from build123d import *

# Parameters (mm, degrees)
BOSS_EXTRUDE1_DEPTH = 76.2
CUT_EXTRUDE1_DEPTH  = 10
SKETCH4_R           = 10
SKETCH4_R_2         = 12.7
CUT_EXTRUDE2_DEPTH  = 10


with BuildPart() as part:
    # Sketch2 → Boss-Extrude1 (new, symmetric)
    with BuildSketch(Plane.XY):
        with BuildLine():
            Line((-38.1, 0), (38.1, 0))
            Line((38.1, 0), (38.1, 101.6))
            Line((38.1, 101.6), (34.925, 101.6))
            ThreePointArc((34.925, 101.6), (32.67993597, 100.67006403), (31.75, 98.425))
            Line((31.75, 98.425), (31.75, 9.525))
            ThreePointArc((31.75, 9.525), (30.82006403, 7.27993597), (28.575, 6.35))
            Line((28.575, 6.35), (-34.925, 6.35))
            ThreePointArc((-34.925, 6.35), (-37.17006403, 5.42006403), (-38.1, 3.175))
            Line((-38.1, 3.175), (-38.1, 0))
        make_face()
    extrude(amount=BOSS_EXTRUDE1_DEPTH, both=True)

    # Sketch3 → Cut-Extrude1 (cut)
    with BuildSketch(Plane(origin=(38.1, 0, 0), x_dir=(0, 0, -1), z_dir=(1, 0, 0))):
        with BuildLine():
            Line((-28.25, 88.9), (-28.25, 38.1))
            ThreePointArc((-28.25, 38.1), (-31.75, 34.6), (-35.25, 38.1))
            Line((-35.25, 38.1), (-35.25, 88.9))
            ThreePointArc((-35.25, 88.9), (-31.75, 92.4), (-28.25, 88.9))
        make_face()
        with BuildLine():
            Line((28.25, 88.9), (28.25, 38.1))
            ThreePointArc((28.25, 38.1), (31.75, 34.6), (35.25, 38.1))
            Line((35.25, 38.1), (35.25, 88.9))
            ThreePointArc((35.25, 88.9), (31.75, 92.4), (28.25, 88.9))
        make_face()
        with BuildLine():
            Line((3.5, 88.9), (3.5, 38.1))
            ThreePointArc((3.5, 38.1), (0, 34.6), (-3.5, 38.1))
            Line((-3.5, 38.1), (-3.5, 88.9))
            ThreePointArc((-3.5, 88.9), (0, 92.4), (3.5, 88.9))
        make_face()
    extrude(amount=-CUT_EXTRUDE1_DEPTH, mode=Mode.SUBTRACT)

    # Sketch4 → Cut-Extrude2 (cut)
    with BuildSketch(Plane.XZ):
        with Locations(Location((0, 0, 0), (0, 0, 270))):
            Circle(SKETCH4_R)
        with Locations(Location((0, 52.5, 0), (0, 0, 270))):
            Circle(SKETCH4_R_2)
        with Locations(Location((0, -52.5, 0), (0, 0, 270))):
            Circle(SKETCH4_R_2)
    extrude(amount=-CUT_EXTRUDE2_DEPTH, mode=Mode.SUBTRACT)


solid = part.part
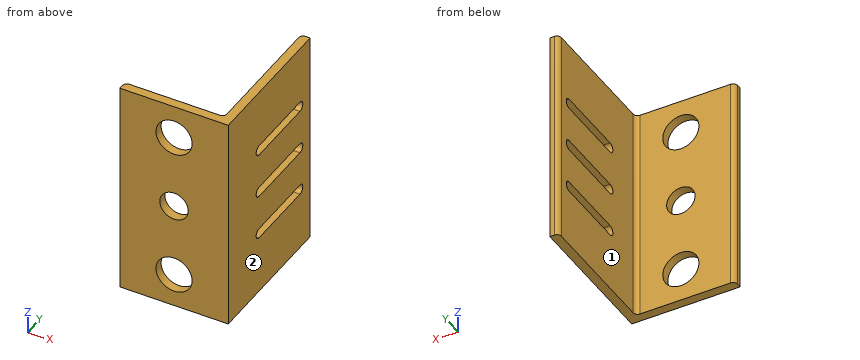
CAD build for the part. Positions are in the model's coordinates, mm. Face numbers are marked on the shaded views. A direction names the side the tool comes from. Give positions to 0.01 mm unless a question says otherwise; leave off trailing zeros. Write each loop counter-clockwise with the first axis right and the second up, starting at its lowest first coordinate (ties: lowest second). Pieces come first, ordered by that corner, then holes. Notation, with made-up numbers: M 80.5,-19 L 114.5,-19 A17 cw 114.5,-12 Z; hole C -15.75,-39 d4. An arc over 180 degrees is marked long. Put each result on its own line as item: value. Start each with the question number.
(1) Which spindle directions (+Z, -Z, +X, -X, +Y, -Y) get a long thin tool onto all of the face, cutting with end or side? Do the marked faces 1 and 2. Say none if no direction does.
(2) Band-saw the part on A-A, the plane x = 0. Write the cut outline in (y, z), and give its area (3 significant figures).
(3) Band-saw the part on B-B, the plane z = -6. Write the cut outline in (x, y) (3 decimals), and give its area (3 significant figures).
(4) Flat gauge pins, fed straight in: pin 1 Ø4 at (x, z) = (4, 24.5) entering from +Y; pin 2 Ø23 at (x, z) = (0, -52.5) entering from -Y; pin 3 Ø1.5 at (y, z) = (24, -32.5) entering from -X. Where does each tip first touch, or does it go through?
(5) Band-saw the part on D-D, the plane z = -31.75. Write the cut outline in (x, y) (3 decimals), and give its area (3 significant figures).
(6) Band-saw the part on C-C, the plane y = 87. Write the cut outline in (x, z).
(7) Probe L1, parallel to X at y = 3, z = 52; L2, parallel to Y at x = 13.5, z = -18.5; L3, parallel to X at y = 46, z = 44.5. List the from-to ranges inside material, lowest first.
Response values:
1. face 1: +Z, -Z, -X, +Y
1. face 2: +Z, -Z, +X, +Y, -Y
2. outline: M 0,-76.2 L 6.35,-76.2 L 6.35,-65.2 L 0,-65.2 Z; M 0,-39.8 L 6.35,-39.8 L 6.35,-10 L 0,-10 Z; M 0,10 L 6.35,10 L 6.35,39.8 L 0,39.8 Z; M 0,65.2 L 6.35,65.2 L 6.35,76.2 L 0,76.2 Z
2. area: 518 mm2
3. outline: M -38.1,0 L -8,0 L -8,6.35 L -34.925,6.35 A3.175 ccw -38.1,3.175 Z; M 8,0 L 38.1,0 L 38.1,101.6 L 34.925,101.6 A3.175 ccw 31.75,98.425 L 31.75,9.525 A3.175 cw 28.575,6.35 L 8,6.35 Z
3. area: 985 mm2
4. pin 1: stops at y = 6.35
4. pin 2: passes through
4. pin 3: stops at x = 31.75
5. outline: M -38.1,0 L 38.1,0 L 38.1,34.6 L 31.75,34.6 L 31.75,9.525 A3.175 cw 28.575,6.35 L -34.925,6.35 A3.175 ccw -38.1,3.175 Z; M 31.75,92.4 L 38.1,92.4 L 38.1,101.6 L 34.925,101.6 A3.175 ccw 31.75,98.425 Z
5. area: 720 mm2
6. outline: M 31.75,-76.2 L 38.1,-76.2 L 38.1,-35.25 L 31.75,-35.25 Z; M 31.75,-28.25 L 38.1,-28.25 L 38.1,-3.5 L 31.75,-3.5 Z; M 31.75,3.5 L 38.1,3.5 L 38.1,28.25 L 31.75,28.25 Z; M 31.75,35.25 L 38.1,35.25 L 38.1,76.2 L 31.75,76.2 Z
7. L1: x = -38.1 to -12.69, 12.69 to 38.1
7. L2: y = 0 to 6.35
7. L3: x = 31.75 to 38.1
